Part model, mm, in its own coordinate system. Coordinates: 2 decimals unless noted, no trailing zeros. Loops run counter-clockwise (first coordinate to the right, second up) from the corner with the lowest first, then second, coordinate; pieces in that order, holes last. Notation, with made-up numbers: (-35.5, 69) - (-4.5, 69) arc R26 ccw to (-4.5, 85) - close; hole circle Ø1 at (56.5, -17). An arc over 180 degrees is marked (long way). Use a Markdown table: item, result. Add a question column.
1) Pull direction X, two halves, no side cores. Call faces 1 (the face through (0, 10, 2)), 2 (the face through (99.408, 10.601, 2.535)), 3 (the face through (123, 30, 0)): +X half, -X half, draft (parallel to the pull), parting line (faces both ways), or undercut.
2) Drop flat-ended pins along their axis: P1, Ø3.5, axis at x = 37.5, y = 30, coming from the -Z side; P2, Ø1, axis at y = 32.5, z = 1.5, coming from the -X side. Give the stop position or say it passes through.
3) Band-saw the part on A-A (z = 1.1). Give the number of separate pieces and of enclosed holes in the cut face, plus the area to 3 significant figures.
4) Probe probe 1 along Y at (x, z) = (37.5, 4.05); probe 2 along Y at (x, z) = (152.5, 2.3); probe 3 along X at (y, z) = (39, 4.4). List the from-to ranges inside material, lowest first. Write a range as [from, to].
5) Band-saw the part on C-C (y = 25.5). Give the cut face in (x, z) (3 decimals).
6) Band-saw the part on B-B (y = 42). Give the cut face in (x, z), plus the area to 3 significant figures.
from build123d import *

# Parameters (mm, degrees)
ESQUISSE1_W                  = 250
ESQUISSE1_H                  = 60
BOSS_EXTRU_1_DEPTH           = 5
ESQUISSE2_R                  = 2
ENL_V_MAT_EXTRU_1_DEPTH      = 5
ENL_V_MAT_EXTRU_2_DEPTH      = 258.147817412
ENL_V_MAT_EXTRU_2_DEPTH_BACK = 258.147817412


with BuildPart() as part:
    # Esquisse1 → Boss.-Extru.1 (new body)
    with BuildSketch(Plane.XY):
        with Locations((125, 30)):
            Rectangle(ESQUISSE1_W, ESQUISSE1_H)
    extrude(amount=BOSS_EXTRU_1_DEPTH)

    # Esquisse2 → Enlèv. mat.-Extru.1 (cut)
    with BuildSketch(Plane.XY.offset(5)):
        with Locations((37.5, 10)):
            Circle(ESQUISSE2_R)
        with Locations((97.5, 10)):
            Circle(ESQUISSE2_R)
        with Locations(Location((152.5, 10, 0), (0, 0, 180))):
            Circle(ESQUISSE2_R)
        with Locations(Location((212.5, 10, 0), (0, 0, 180))):
            Circle(ESQUISSE2_R)
        with Locations((240, 50)):
            Circle(ESQUISSE2_R)
        with Locations((240, 30)):
            Circle(ESQUISSE2_R)
        with Locations((37.5, 30)):
            Circle(ESQUISSE2_R)
        with Locations((37.5, 50)):
            Circle(ESQUISSE2_R)
        with Locations(Location((97.5, 50, 0), (0, 0, 180))):
            Circle(ESQUISSE2_R)
        with Locations(Location((97.5, 30, 0), (0, 0, 180))):
            Circle(ESQUISSE2_R)
    extrude(amount=-ENL_V_MAT_EXTRU_1_DEPTH, mode=Mode.SUBTRACT)

    # Esquisse3 → Enlèv. mat.-Extru.2 (cut, two sides: drawn at the far end of the back side and taken through both)
    with BuildSketch(Plane.XY.offset(5).offset(-ENL_V_MAT_EXTRU_2_DEPTH_BACK)):
        Polygon((0, 20), (30, 60), (0, 60), align=None)
    extrude(amount=ENL_V_MAT_EXTRU_2_DEPTH + ENL_V_MAT_EXTRU_2_DEPTH_BACK, mode=Mode.SUBTRACT)


solid = part.part
Answer block:
| question | item | result |
|---|---|---|
| 1 | face 1 | -X half |
| 1 | face 2 | undercut |
| 1 | face 3 | draft |
| 2 | P1 | through |
| 2 | P2 | x = 9 |
| 3 | separate pieces | 1 |
| 3 | enclosed holes | 10 |
| 3 | area | 14,300 mm2 |
| 4 | probe 1 | [0, 8], [12, 28], [32, 48], [52, 60] |
| 4 | probe 2 | [0, 8], [12, 60] |
| 4 | probe 3 | [14.25, 250] |
| 5 | outline | (4.125, 0) - (250, 0) - (250, 5) - (4.125, 5) - close |
| 6 | outline | (16.5, 0) - (250, 0) - (250, 5) - (16.5, 5) - close |
| 6 | area | 1,170 mm2 |
